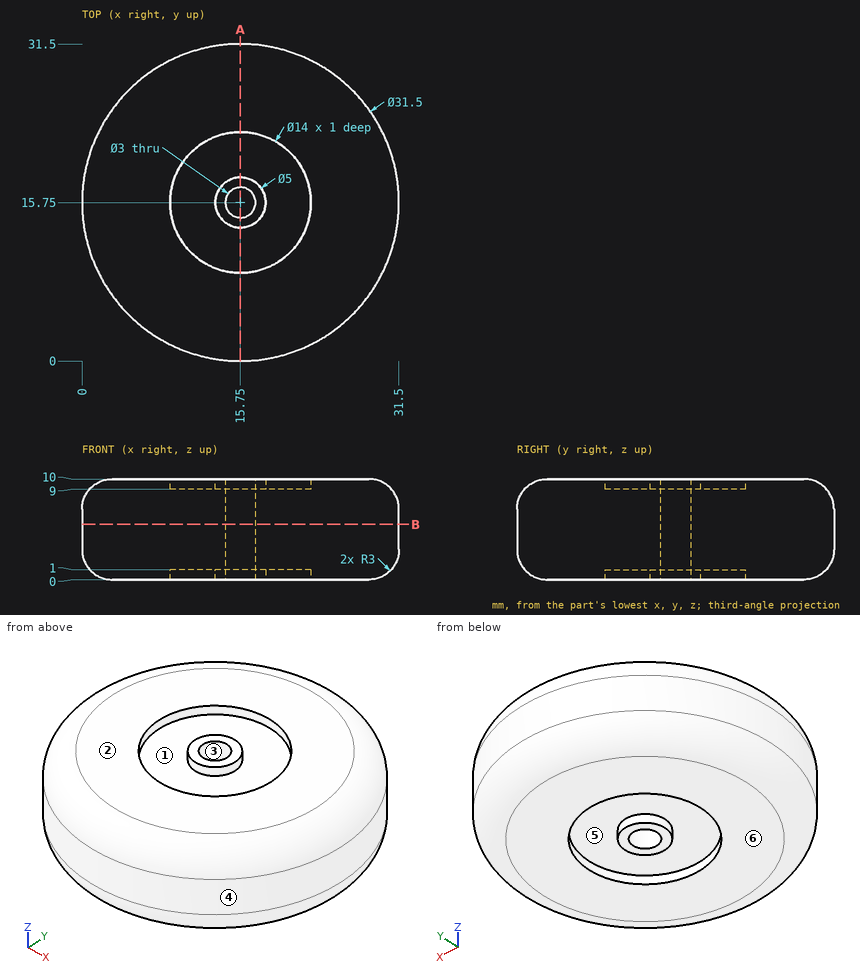
Geometry check sheet. Reference: drawing and pictorial views, mm from the part's lowest x, y, z. A direction names the side the tool comes from. Give positions to 0.01 mm unless a question says otherwise; leave off trailing zeros. Loops run counter-clockwise (first coordinate to the right, second up) from the corner with the lowest first, then second, coordinate; pieces in that order, holes last. Notation, with made-up numbers: (-5.5, -17) - (40.5, -17) arc R36 ccw to (40.5, 17) - close; hole circle Ø2 at (49.25, -39.5). An arc over 180 degrees is marked (long way). Use CSV: the item, a comma, the result in double quotes. Start each with the question number.
Q1. Section check A-A, the plane x = 15.75. Record the cut outline in (y, z), and give its area (3 significant figures).
Q2. Go/stop test with flat-tipped pins: pin 1 Ø5 at (y, z) = (19.5, 6.5) entering from +X; pin 2 Ø3 at (y, z) = (11, 4.5) entering from -X; pin 3 Ø6 at (x, z) = (9, 1.5) entering from +Y; pin 4 Ø1.8 at (x, y) = (15.75, 15.75) entering from +Z. Record where each tip stops, or that it passes through.
Q3. Scan lines: probe 1 along Y at (x, z) = (15.75, 0.75); probe 2 along Y at (x, z) = (15.75, 6); probe 3 along Y at (x, z) = (15.75, 0.85). Record each from-to range of solid material in increasing order. Write a range as from..to.
Q4. Access from +Z, -Z, +X, -X, +Y, -Y to the whole of each face (thin tool, end or side, straight path). Record for the marked faces 1 and 2.
Q5. Section check B-B, the plane z = 5.5. Record the cut outline in (x, y).
Q6. Release check for a two-part mould opening along X. For the marked faces 3, 4, 5 and 6 record: +X half, -X half, draft (parallel to the pull), parting line (faces both ways), or undercut.
Findings below:
1,outline,"(0, 3) arc R3 ccw to (3, 0) - (8.75, 0) - (8.75, 1) - (13.25, 1) - (13.25, 0) - (14.25, 0) - (14.25, 10) - (13.25, 10) - (13.25, 9) - (8.75, 9) - (8.75, 10) - (3, 10) arc R3 ccw to (0, 7) - close; (17.25, 0) - (18.25, 0) - (18.25, 1) - (22.75, 1) - (22.75, 0) - (28.5, 0) arc R3 ccw to (31.5, 3) - (31.5, 7) arc R3 ccw to (28.5, 10) - (22.75, 10) - (22.75, 9) - (18.25, 9) - (18.25, 10) - (17.25, 10) - close"
1,area,"259 mm^2"
2,pin 1,"stops at x = 31.45"
2,pin 2,"stops at x = 0.34"
2,pin 3,"stops at y = 30.97"
2,pin 4,"passes through"
3,probe 1,"y = 1.02..8.75, 13.25..14.25, 17.25..18.25, 22.75..30.48"
3,probe 2,"y = 0..14.25, 17.25..31.5"
3,probe 3,"y = 0.91..8.75, 13.25..14.25, 17.25..18.25, 22.75..30.59"
4,face 1,"+Z"
4,face 2,"+Z, +X, -X, +Y, -Y"
5,outline,"circle Ø31.5 at (15.75, 15.75); hole circle Ø3 at (15.75, 15.75)"
6,face 3,"undercut"
6,face 4,"parting line"
6,face 5,"undercut"
6,face 6,"draft"
